from build123d import *

# Parameters (mm, degrees)
F0_R     = 1.25
F0_W     = 51
F0_H     = 5
F1_DEPTH = 2
F2_DEPTH = 15


with BuildPart() as f1:
    # F0 (on Top) → F1 (new body)
    with BuildSketch(Plane.XY):
        with BuildLine():
            ThreePointArc((31.101435, 12), (30.222755, 14.12132), (28.101435, 15))
            Line((28.101435, 15), (-30.898565, 15))
            ThreePointArc((-30.898565, 15), (-33.019886, 14.12132), (-33.898565, 12))
            Line((-33.898565, 12), (-33.898565, -12))
            ThreePointArc((-33.898565, -12), (-33.019886, -14.12132), (-30.898565, -15))
            Line((-30.898565, -15), (28.101435, -15))
            ThreePointArc((28.101435, -15), (30.222755, -14.12132), (31.101435, -12))
            Line((31.101435, -12), (31.101435, 12))
        make_face()
        with Locations((-30.398565, -11.5)):
            Circle(F0_R, mode=Mode.SUBTRACT)
        with Locations((27.601435, -11.5)):
            Circle(F0_R, mode=Mode.SUBTRACT)
        with Locations((-30.398565, 11.5)):
            Circle(F0_R, mode=Mode.SUBTRACT)
        with Locations((-1.398565, 11.2)):
            Rectangle(F0_W, F0_H, mode=Mode.SUBTRACT)
        with Locations((27.601435, 11.5)):
            Circle(F0_R, mode=Mode.SUBTRACT)
        with Locations((-1.398565, 11.2)):
            Rectangle(F0_W, F0_H)
    extrude(amount=F1_DEPTH)

    # F0 (on Top) → F2 (join)
    with BuildSketch(Plane.XY):
        with Locations((-1.398565, 11.2)):
            Rectangle(F0_W, F0_H)
    extrude(amount=F2_DEPTH)


solid = f1.part
Here's how the part is built. I have some questions about the finished solid (model axes, mm). A direction names the side the tool comes from. Coordinates: 2 decimals unless noted, no trailing zeros. Write each loop counter-clockwise with the first axis right and the second up, starting at its lowest first coordinate (ties: lowest second). Pieces come first, ordered by that corner, then holes.
Item 1: Will these pins go through, and if not, where does the flat tip stop? pin 1 (4 mm diameter, centred on y = 11, z = 10.5, fed in from -X); pin 2 (1.5 mm diameter, centred on y = 11.5, z = 8, fed in from +X); pin 3 (1.5 mm diameter, centred on x = 17.5, z = 13.5, fed in from +Y); pin 4 (4 mm diameter, centred on x = 27.6, y = -11.5, fed in from -Z).
Item 2: I want a section at B-B on z = 7. Write out the boundary of the cut face in (x, y), and give its area (3 significant figures).
Item 3: If we mould it in two halves opening along Y, with no side actions, what happens to faces 1 (the flat face through (-2, 8.7, 8)), 2 (the cylindrical face through (28.794, 11.875, 0.986)), 3 (the flat face through (24.101, 11, 8))? For each: +Y half, -Y half, draft (parallel to the pull), parting line (faces both ways), or undercut.
Item 4: I want a section at C-C on y = -5.5. Write out the boundary of the cut face in (x, z).
Item 5: On a 3-axis mill with a long thin cutter (end or side, diameter ignored), from which of +Z, -Z, +X, -X, +Y, -Y can I reach the whole of each face in a straight line? I mean faces 4 (the flat face through (-26.899, 11, 8)), 5 (the flat face through (-2, 13.7, 8)), 6 (the cylindrical face through (-29.206, -11.125, 0.986)). Say none if no direction works.
Item 6: I want a section at A-A on x = -15. Write out the boundary of the cut face in (y, z), and give its area (3 significant figures).
Item 7: If I drill on line 1 (Y direction, x = 15, z = 10.5); line 2 (Z direction, x = 10, y = -3); line 3 (X direction, y = 13, z = 4), over which ranges is the centre line in solid material (lowest first)?
Findings below:
1. pin 1: stops at x = -26.9
1. pin 2: stops at x = 24.1
1. pin 3: stops at y = 13.7
1. pin 4: stops at z = 0
2. outline: (-26.9, 8.7) - (24.1, 8.7) - (24.1, 13.7) - (-26.9, 13.7) - close
2. area: 255 mm2
3. face 1: -Y half
3. face 2: undercut
3. face 3: draft
4. outline: (-33.9, 0) - (31.1, 0) - (31.1, 2) - (-33.9, 2) - close
5. face 4: +Z, -X, +Y, -Y
5. face 5: +Z, +X, -X, +Y
5. face 6: +Z, -Z
6. outline: (-15, 0) - (15, 0) - (15, 2) - (13.7, 2) - (13.7, 15) - (8.7, 15) - (8.7, 2) - (-15, 2) - close
6. area: 125 mm2
7. line 1: y = 8.7 to 13.7
7. line 2: z = 0 to 2
7. line 3: x = -26.9 to 24.1
